Check sheet for the modelled part. Datum: model origin and axes. Units: mm. Face numbers are marked on the shaded views. Round coordinates to 2 decimals unless told otherwise and drop trailing zeros.
(1) Depth check by flat-ended pin: pin 1 (9 mm diameter, centred on x = -15.875, y = 0, fed in from -Z) (3 decimals); pin 2 (1 mm diameter, centred on y = 10, z = -1.5, fed in from +X); pin 3 (5 mm diameter, centred on x = 4, y = -3.5, fed in from +Z); pin 4 (5 mm diameter, centred on x = 0, y = -15.875, fed in from +Z). Enter the tip coordinate at first touch or a pass-through.
(2) Thickness scan on probe 1 along Y at (x, z) = (0, -2.1) (1 decimal); probe 2 along Y at (x, z) = (0, -0.6) (1 decimal); probe 3 along X at (y, z) = (-0.5, 1.5). Record the ranges inside material, lowest first.
(3) Mould release check, pull along Y, two halves, no side actions. Record for the marked faces 1, 2 and 3: released by +Y, released by -Y, zero draft, split by the parting line, or undercut.
(4) Sectioned sample at A-A, the plane x = 0. Count the separate pieces of the cut face and the enclosed holes in it, and give its area (3 significant figures).
Autodesk Inventor part; units mm, degrees
ref_plane "YZ Plane" through (0, 0, 0) normal (1, 0, 0) x (0, 1, 0)
ref_plane "XZ Plane" through (0, 0, 0) normal (0, 1, 0) x (-1, 0, 0)
ref_plane "XY Plane" through (0, 0, 0) normal (0, 0, 1) x (1, 0, 0)
sketch "Sketch1" plane through (0, 0, 0) normal (0, 0, 1) x (1, 0, 0)
  circle A0 centre (0, 0) radius 9.525
  line L0 (0, 0) -> (0, 15.875)
  circle A1 centre (0, 15.875) radius 1.5875
  circle A2 centre (-15.875, 0) radius 1.5875
  circle A3 centre (0, -15.875) radius 1.5875
  circle A4 centre (15.875, 0) radius 1.5875
  circle A5 centre (0, 0) radius 20.6375
  dimension "d0" = 19.05
  dimension "d1" = 15.875
  dimension "d2" = 3.175
  dimension "d5" = 360
  dimension "d7" = 41.275
extrude "Extrusion1" add sketch "Sketch1" against normal blind 3.175
chamfer "Chamfer1" distance 1.27 angle 45 4 edges at (-1.5875, 15.875, 0) (14.2875, 0, 0) (-1.5875, -15.875, 0) (-17.4625, 0, 0)
sketch "Sketch4" plane through (0, 0, 0) normal (0, 0, 1) x (1, 0, 0)
  circle A0 centre (0, -15.875) radius 2.8575
  circle A1 centre (0, 15.875) radius 2.8575
  circle A2 centre (0, 0) radius 9.525
  circle A3 centre (0, 0) radius 20.6375
  circle A4 centre (15.875, 0) radius 2.8575
  circle A5 centre (-15.875, 0) radius 2.8575
extrude "Extrusion3" add sketch "Sketch4" along normal blind 2.032
sketch "Sketch5" plane through (0, 0, 2.032) normal (0, 0, 1) x (1, 0, 0)
  circle A0 centre (0, 0) radius 12.065
  dimension "d17" = 24.13
extrude "Extrusion4" cut sketch "Sketch5" against normal blind 3.81
sketch "Sketch6" plane through (0, 0, 2.032) normal (0, 0, 1) x (1, 0, 0)
  circle A0 centre (0, 0) radius 19.2405
  circle A1 centre (0, 0) radius 20.0025
  dimension "d20" = 38.481
  dimension "d21" = 40.005
extrude "Extrusion5" add sketch "Sketch6" along normal blind 1.27
chamfer "Chamfer2" distance 0.762 distance2 1.27 1 edges at (-20.0025, 0, 3.302) measured on face at (19.3684, -3.1305, 3.302)
chamfer "Chamfer3" distance 0.635 distance2 1.016 1 edges at (-20.6375, 0, 2.032) measured on face at (20.0322, -3.2419, 2.032)
properties part number "RadialBearingMountCover" material "ABS Plastic"
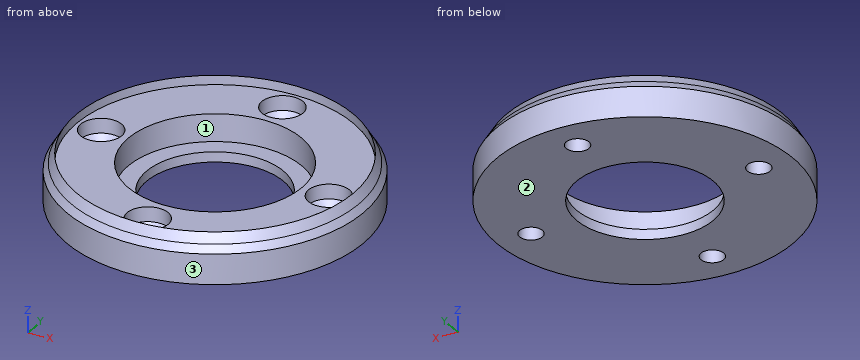
Derived:
1. pin 1: stops at z = -3.175
1. pin 2: stops at x = 18.32
1. pin 3: passes through
1. pin 4: stops at z = -0.36
2. probe 1: y = -20.6 to -17.5, -14.3 to -9.5, 9.5 to 14.3, 17.5 to 20.6
2. probe 2: y = -20.6 to -18.1, -13.6 to -12.1, 12.1 to 13.6, 18.1 to 20.6
2. probe 3: x = -20.33 to -18.69, -13.06 to -12.05, 12.05 to 13.06, 18.69 to 20.33
3. face 1: undercut
3. face 2: zero draft
3. face 3: split by the parting line
4. separate pieces: 4
4. enclosed holes: 0
4. area: 50.1 mm2
